from build123d import *

# Parameters (mm, degrees)
SKETCH2_W           = 76.2
SKETCH2_H           = 82.55
BOSS_EXTRUDE1_DEPTH = 4.7752
SKETCH3_W           = 38.1
SKETCH3_H           = 4.7752
SKETCH3_W_2         = 25.4
CUT_EXTRUDE1_DEPTH  = 4.7752
SKETCH4_W           = 4.7752
SKETCH4_H           = 19.05
SKETCH4_H_2         = 12.7
SKETCH4_H_3         = 20.6248
CUT_EXTRUDE2_DEPTH  = 4.7752
SKETCH5_W           = 4.7752
SKETCH5_H           = 4.7752
SKETCH5_H_2         = 12.7
SKETCH5_H_3         = 6.35
CUT_EXTRUDE3_DEPTH  = 4.7752


with BuildPart() as part:
    # Sketch2 → Boss-Extrude1 (new body)
    with BuildSketch(Plane.XY):
        with Locations((38.1, 41.275)):
            Rectangle(SKETCH2_W, SKETCH2_H)
    extrude(amount=BOSS_EXTRUDE1_DEPTH)

    # Sketch3 → Cut-Extrude1 (cut)
    with BuildSketch(Plane.XY.offset(4.7752)):
        with Locations((19.05, 2.3876)):
            Rectangle(SKETCH3_W, SKETCH3_H)
        with Locations((63.5, 2.3876)):
            Rectangle(SKETCH3_W_2, SKETCH3_H)
    extrude(amount=-CUT_EXTRUDE1_DEPTH, mode=Mode.SUBTRACT)

    # Sketch4 → Cut-Extrude2 (cut)
    with BuildSketch(Plane.XY.offset(4.7752)):
        with Locations((2.3876, 73.025)):
            Rectangle(SKETCH4_W, SKETCH4_H)
        with Locations((2.3876, 44.45)):
            Rectangle(SKETCH4_W, SKETCH4_H_2)
        with Locations((2.3876, 15.0876)):
            Rectangle(SKETCH4_W, SKETCH4_H_3)
    extrude(amount=-CUT_EXTRUDE2_DEPTH, mode=Mode.SUBTRACT)

    # Sketch5 → Cut-Extrude3 (cut)
    with BuildSketch(Plane.XY.offset(4.7752)):
        with Locations((73.8124, 7.1628)):
            Rectangle(SKETCH5_W, SKETCH5_H)
        with Locations((73.8124, 31.75)):
            Rectangle(SKETCH5_W, SKETCH5_H_2)
        with Locations((73.8124, 57.15)):
            Rectangle(SKETCH5_W, SKETCH5_H_2)
        with Locations((73.8124, 79.375)):
            Rectangle(SKETCH5_W, SKETCH5_H_3)
    extrude(amount=-CUT_EXTRUDE3_DEPTH, mode=Mode.SUBTRACT)


solid = part.part
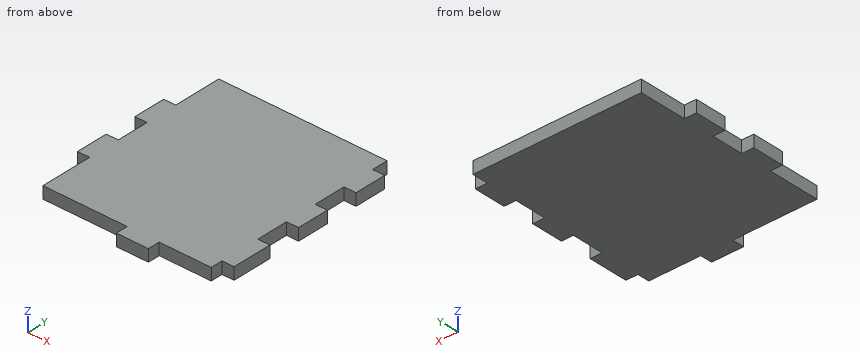
Geometry: final body of the model. Coordinates: model frame, mm. Give positions to 0.01 mm unless a question says otherwise; leave off trailing zeros. Write each loop counter-clockwise with the first axis right and the second up, starting at its lowest first coordinate (ties: lowest second). Pieces come first, ordered by that corner, then holes. Notation, with made-up numbers: (2.5, 15.25) -> (52.5, 15.25) arc R16 ccw to (52.5, 45.25) -> close; hole circle Ø2 at (64.25, 34.25). An arc over 180 degrees is marked (long way). Answer as a JSON object with one key per item and string values.
1. Cut plane A-A on z = 1.4. Output: boundary loops of the cut face in (x, y), and give its area (3 significant figures).
Ans:
{"outline": "(0, 25.4) -> (4.78, 25.4) -> (4.78, 4.78) -> (38.1, 4.78) -> (38.1, 0) -> (50.8, 0) -> (50.8, 4.78) -> (71.42, 4.78) -> (71.42, 9.55) -> (76.2, 9.55) -> (76.2, 25.4) -> (71.42, 25.4) -> (71.42, 38.1) -> (76.2, 38.1) -> (76.2, 50.8) -> (71.42, 50.8) -> (71.42, 63.5) -> (76.2, 63.5) -> (76.2, 76.2) -> (71.42, 76.2) -> (71.42, 82.55) -> (4.78, 82.55) -> (4.78, 63.5) -> (0, 63.5) -> (0, 50.8) -> (4.78, 50.8) -> (4.78, 38.1) -> (0, 38.1) -> close", "area": "5,560 mm^2"}
2. Cut plane C-C on x = 11. Output: boundary loops of the cut face in (y, z), and give its area (3 significant figures).
Ans:
{"outline": "(4.78, 0) -> (82.55, 0) -> (82.55, 4.78) -> (4.78, 4.78) -> close", "area": "371 mm^2"}
3. Contact query for flat-ended pins moving along their axis: pin 1 (1.4 mm diameter, centred on x = 2, z = 2.5, fed in from -Y); pin 2 (2 mm diameter, centred on x = 59, z = 2, fed in from -Y); pin 3 (2.5 mm diameter, centred on y = 80, z = 2.5, fed in from +X); pin 4 (4 mm diameter, centred on x = 11.5, y = 35.5, fed in from -Z). Output: stop coordinate, or through.
Ans:
{"pin 1": "stops at y = 25.4", "pin 2": "stops at y = 4.78", "pin 3": "stops at x = 71.42", "pin 4": "stops at z = 0"}
4. Cut plane B-B on y = 6. Output: boundary loops of the cut face in (x, z).
Ans:
{"outline": "(4.78, 0) -> (71.42, 0) -> (71.42, 4.78) -> (4.78, 4.78) -> close"}
5. Ray query, probe 1 along Y at (x, z) = (33.5, 4.55); probe 2 along X at (y, z) = (76, 4.15); probe 3 along X at (y, z) = (29, 2.1). Return the intervals inside material, ascending. Write a range as from..to.
Ans:
{"probe 1": "y = 4.78..82.55", "probe 2": "x = 4.78..76.2", "probe 3": "x = 0..71.42"}
